The model under review builds one solid part; all positions refer to its coordinate system, in mm. A direction names the side the tool comes from. Round coordinates to 2 decimals unless told otherwise and drop trailing zeros. Loops run counter-clockwise (first coordinate to the right, second up) from the corner with the lowest first, then second, coordinate; pieces in that order, holes last. Notation, with made-up numbers: (-40, 5.25) -> (-1, 5.25) arc R23 ccw to (-1, 31.25) -> close; hole circle Ø6 at (56.5, 88). An arc over 180 degrees is marked (long way). Use a Markdown table: item, result. Add a question column.
1) Wall thickness on probe 1 along Z at (x, y) = (55, -17); probe 2 along Z at (x, y) = (34, -4.5); probe 3 along X at (y, z) = (-11.5, -120.65): over which ranges is each line inside the solid? List them lowest first.
2) Insertion check: pin 1 (5 mm diameter, centred on y = -13.5, z = -118, fed in from +X); pin 2 (1.5 mm diameter, centred on x = 8, z = -73, fed in from +Y); pin 3 (1 mm diameter, centred on x = 33, z = -109.5, fed in from -Y); pin 4 (8 mm diameter, centred on x = 8.5, z = -101, fed in from -Y). Each pin has a flat end and moves straight along its axis. Give the tip position at first contact, or say it passes through.
3) For faces 1 (the flat face through (36, -23, -137.16)), 2 (the flat face through (38, -23, -7.62)), 3 (the flat face through (38.5, 5.08, -53.3)), list the 3-axis set-ups (+Z, -Z, +X, -X, +Y, -Y) from which the entire face can be reached by the end or side of a thin tool; tool diameter is ignored.
4) Consider section A-A on z = -55.88. Give the boundary of the cut face in (x, y), plus the area to 3 significant figures.
5) Consider section C-C on z = -78.5. Give the boundary of the cut face in (x, y), plus the area to 3 significant figures.
6) Mouldability with a two-part tool opening along X and no side actions: class faces 4 (the cylindrical face through (41.156, 6.368, -61.832)), 5 (the flat face through (35, -23, 0)), 6 (the flat face through (0, -20, -69)) as released by +X, released by -X, zero draft, split by the parting line, or undercut.
7) Consider section D-D on x = 51. Give the boundary of the cut face in (y, z).
8) Consider section B-B on y = -24.13. Give the boundary of the cut face in (x, z).
from build123d import *

# Parameters (mm, degrees)
SKETCH1_W           = 58.42
SKETCH1_H           = 137.16
BOSS_EXTRUDE1_DEPTH = 7.62
SKETCH2_R           = 6.35
SKETCH2_R_2         = 4.826
BOSS_EXTRUDE2_DEPTH = 35.56
BOSS_EXTRUDE3_DEPTH = 35.56
FILLET1_R           = 19.05
FILLET2_R           = 12.7
BOSS_EXTRUDE4_DEPTH = 5.08
SKETCH7_R           = 7.5
CUT_EXTRUDE1_DEPTH  = 158.192964219
CUT_EXTRUDE2_START  = -5.08
SKETCH8_R           = 11
SKETCH8_R_2         = 7.5
CUT_EXTRUDE2_DEPTH  = 5.08
FILLET3_R           = 10.16
CUT_EXTRUDE3_REACH  = 157.273
SKETCH9_R           = 8.5


with BuildPart() as part:
    # Sketch1 → Boss-Extrude1 (new body)
    with BuildSketch(Plane(origin=(0, 0, 0), x_dir=(1, 0, 0), z_dir=(0, 1, 0))):
        with Locations((29.21, 68.58)):
            Rectangle(SKETCH1_W, SKETCH1_H)
    extrude(amount=BOSS_EXTRUDE1_DEPTH)

    # Sketch2 → Boss-Extrude2 (add)
    # profile 1 of 2: a face of its own
    with BuildSketch(Plane.XZ):
        with Locations(Location((28.448, -120.65, 0), (0, 0, 270))):
            Circle(SKETCH2_R)
        with Locations(Location((28.448, -120.65, 0), (0, 0, 270))):
            Circle(SKETCH2_R_2, mode=Mode.SUBTRACT)
    # profile 2 of 2: a face of its own
    with BuildSketch(Plane.XZ):
        with Locations(Location((28.448, -15.24, 0), (0, 0, 270))):
            Circle(SKETCH2_R)
        with Locations(Location((28.448, -15.24, 0), (0, 0, 270))):
            Circle(SKETCH2_R_2, mode=Mode.SUBTRACT)
    extrude(amount=BOSS_EXTRUDE2_DEPTH)

    # Sketch3 → Boss-Extrude3 (add)
    with BuildSketch(Plane.XZ):
        Polygon((58.42, -137.16), (0, -137.16), (0, 0), (58.42, 0), (58.42, -7.62), (7.62, -7.62), (7.62, -129.54), (58.42, -129.54), align=None)
    extrude(amount=BOSS_EXTRUDE3_DEPTH)

    # Fillet1
    fillet1_edges = [part.edges().sort_by_distance(p)[0] for p in [
        (29.21, 7.62, -137.16),
        (29.21, 7.62, 0),
    ]]
    fillet(fillet1_edges, radius=FILLET1_R)

    # Fillet2
    fillet2_edges = [part.edges().sort_by_distance(p)[0] for p in [
        (0, 7.62, -68.58),
        (0, -23.495, 0),
        (0, -23.495, -137.16),
        (0, 2.040384182, -131.580384182),
        (0, 2.040384182, -5.579615818),
    ]]
    fillet(fillet2_edges, radius=FILLET2_R)

    # Sketch4 → Boss-Extrude4 (add)
    with BuildSketch(Plane(origin=(58.42, 0, 0), x_dir=(0, 0, -1), z_dir=(1, 0, 0))):
        with BuildLine():
            Line((10.00175133, 5.334), (127.15824867, 5.334))
            ThreePointArc((127.15824867, 5.334), (122.77627796, 7.039660257), (118.11, 7.62))
            Line((118.11, 7.62), (19.05, 7.62))
            ThreePointArc((19.05, 7.62), (14.38372204, 7.039660257), (10.00175133, 5.334))
        make_face()
    extrude(amount=BOSS_EXTRUDE4_DEPTH)

    # Sketch7 → Cut-Extrude1 (cut, through all)
    with BuildSketch(Plane(origin=(0, 7.62, 0), x_dir=(1, 0, 0), z_dir=(0, 1, 0))):
        with Locations(Location((45.72, 55.88, 0), (0, 0, 270))):
            Circle(SKETCH7_R)
        with Locations(Location((33.02, 35.56, 0), (0, 0, 270))):
            Circle(SKETCH7_R)
    extrude(amount=-CUT_EXTRUDE1_DEPTH, mode=Mode.SUBTRACT)

    # Sketch8 → Cut-Extrude2 (cut)
    # profile 1 of 2: a face of its own
    with BuildSketch(Plane.XZ.offset(CUT_EXTRUDE2_START)):
        with Locations(Location((45.72, -55.88, 0), (0, 0, 270))):
            Circle(SKETCH8_R)
        with Locations(Location((45.72, -55.88, 0), (0, 0, 90))):
            Circle(SKETCH8_R_2, mode=Mode.SUBTRACT)
    # profile 2 of 2: a face of its own
    with BuildSketch(Plane.XZ.offset(CUT_EXTRUDE2_START)):
        with Locations(Location((33.02, -35.56, 0), (0, 0, 270))):
            Circle(SKETCH8_R)
        with Locations(Location((33.02, -35.56, 0), (0, 0, 90))):
            Circle(SKETCH8_R_2, mode=Mode.SUBTRACT)
    extrude(amount=CUT_EXTRUDE2_DEPTH, mode=Mode.SUBTRACT)

    # Fillet3
    # the kernel refuses this fillet: 10.16 mm, written as the material it adds along each edge
    with BuildSketch(Plane(origin=(17.78, -10.16, -119.38), x_dir=(0, 1, 0), z_dir=(-1, 0, 0))) as fillet3_piece_1_section:
        Polygon((0, 0), (FILLET3_R * 1.02, 0), (FILLET3_R * 1.02, FILLET3_R * 1.02), (0, FILLET3_R * 1.02), align=None)
    fillet3_piece_1 = extrude(amount=FILLET3_R * 1.02, mode=Mode.PRIVATE)
    fillet3_piece_1 = fillet3_piece_1 - Plane(origin=(17.78, -10.16, -119.38), x_dir=(0, -0.7071067811865475, 0.7071067811865475), z_dir=(-1, 0, 0)) * Sphere(FILLET3_R, mode=Mode.PRIVATE)
    add(fillet3_piece_1)
    with BuildSketch(Plane(origin=(17.78, -10.16, -17.78), x_dir=(0, 0, 1), z_dir=(-1, 0, 0))) as fillet3_piece_2_section:
        Polygon((0, 0), (FILLET3_R * 1.02, 0), (FILLET3_R * 1.02, FILLET3_R * 1.02), (0, FILLET3_R * 1.02), align=None)
    fillet3_piece_2 = extrude(amount=FILLET3_R * 1.02, mode=Mode.PRIVATE)
    fillet3_piece_2 = fillet3_piece_2 - Plane(origin=(17.78, -10.16, -17.78), x_dir=(0, -0.7071067811865475, -0.7071067811865475), z_dir=(-1, 0, 0)) * Sphere(FILLET3_R, mode=Mode.PRIVATE)
    add(fillet3_piece_2)
    with BuildSketch(Plane(origin=(17.78, 0, -129.54), x_dir=(0, 0, 1), z_dir=(1, 0, 0))) as fillet3_piece_3_section:
        with BuildLine():
            CenterArc((FILLET3_R, FILLET3_R), FILLET3_R, 180, 90)
            Line((0, FILLET3_R), (0, 0))
            Line((0, 0), (FILLET3_R, 0))
        make_face()
    fillet3_piece_3 = extrude(amount=40.64, mode=Mode.PRIVATE)
    fillet3_piece_3 = fillet3_piece_3 - Plane(origin=(28.448, -2.379056343, -120.65), x_dir=(0, 0, -1), z_dir=(0, 1, 0)) * Cylinder(4.826, 122, mode=Mode.PRIVATE)
    add(fillet3_piece_3)
    with BuildSketch(Plane(origin=(7.62, 0, -17.78), x_dir=(1, 0, 0), z_dir=(0, 0, -1))) as fillet3_piece_4:
        with BuildLine():
            CenterArc((FILLET3_R, FILLET3_R), FILLET3_R, 180, 90)
            Line((0, FILLET3_R), (0, 0))
            Line((0, 0), (FILLET3_R, 0))
        make_face()
    extrude(amount=101.6)
    with BuildSketch(Plane(origin=(7.62, -10.16, -129.54), x_dir=(1, 0, 0), z_dir=(0, -1, 0))) as fillet3_piece_5:
        with BuildLine():
            CenterArc((FILLET3_R, FILLET3_R), FILLET3_R, 180, 90)
            Line((0, FILLET3_R), (0, 0))
            Line((0, 0), (FILLET3_R, 0))
        make_face()
    extrude(amount=25.4)
    with BuildSketch(Plane(origin=(58.42, 0, -7.62), x_dir=(0, -1, 0), z_dir=(-1, 0, 0))) as fillet3_piece_6_section:
        with BuildLine():
            CenterArc((FILLET3_R, -FILLET3_R), FILLET3_R, 90, 90)
            Line((0, -FILLET3_R), (0, 0))
            Line((0, 0), (FILLET3_R, 0))
        make_face()
    fillet3_piece_6 = extrude(amount=40.64, mode=Mode.PRIVATE)
    fillet3_piece_6 = fillet3_piece_6 - Plane(origin=(28.448, -2.418481563, -15.24), x_dir=(0, 0, -1), z_dir=(0, 1, 0)) * Cylinder(4.826, 122, mode=Mode.PRIVATE)
    add(fillet3_piece_6)
    with BuildSketch(Plane(origin=(7.62, -10.16, -7.62), x_dir=(1, 0, 0), z_dir=(0, -1, 0))) as fillet3_piece_7:
        with BuildLine():
            CenterArc((FILLET3_R, -FILLET3_R), FILLET3_R, 90, 90)
            Line((0, -FILLET3_R), (0, 0))
            Line((0, 0), (FILLET3_R, 0))
        make_face()
    extrude(amount=25.4)

    # Sketch9 → Cut-Extrude3 (cut, up to next)
    with BuildSketch(Plane.ZY, mode=Mode.PRIVATE) as cut_extrude3_sk1:
        with Locations((-99.06, -24.13)):
            Circle(SKETCH9_R)
    cut_extrude3_tool1 = extrude(cut_extrude3_sk1.sketch, amount=-CUT_EXTRUDE3_REACH, mode=Mode.PRIVATE) & part.part
    add(cut_extrude3_tool1.solids().sort_by_distance((0, -24.13, -99.06))[0], mode=Mode.SUBTRACT)


solid = part.part
Result set:
| question | item | result |
|---|---|---|
| 1 | probe 1 | -137.16 to -129.54, -7.62 to 0 |
| 1 | probe 2 | -135.85 to -127.82, -123.73 to -117.57, -18.32 to -12.16, -9.34 to -1.31 |
| 1 | probe 3 | 0 to 7.7, 22.1 to 23.62, 33.27 to 34.8 |
| 2 | pin 1 | x = 34.8 |
| 2 | pin 2 | y = 6.99 |
| 2 | pin 3 | y = 0 |
| 2 | pin 4 | y = -35.56 |
| 3 | face 1 | -Z, +X, -X, +Y, -Y |
| 3 | face 2 | +X, -Y |
| 3 | face 3 | -Y |
| 4 | outline | (0, -35.56) -> (7.62, -35.56) -> (7.62, -10.16) arc R10.16 cw to (17.78, 0) -> (34.72, 0) -> (34.72, 5.08) -> (38.22, 5.08) -> (38.22, 7.62) -> (12.7, 7.62) arc R12.7 ccw to (0, -5.08) -> close; (53.22, 5.08) -> (56.72, 5.08) -> (56.72, 0) -> (58.42, 0) -> (58.42, 5.33) -> (63.5, 5.33) -> (63.5, 7.62) -> (53.22, 7.62) -> close |
| 4 | area | 565 mm2 |
| 5 | outline | (0, -35.56) -> (7.62, -35.56) -> (7.62, -10.16) arc R10.16 cw to (17.78, 0) -> (58.42, 0) -> (58.42, 5.33) -> (63.5, 5.33) -> (63.5, 7.62) -> (12.7, 7.62) arc R12.7 ccw to (0, -5.08) -> close |
| 5 | area | 715 mm2 |
| 6 | face 4 | undercut |
| 6 | face 5 | zero draft |
| 6 | face 6 | released by -X |
| 7 | outline | (-35.56, -137.16) -> (-11.43, -137.16) arc R19.05 ccw to (7.62, -118.11) -> (7.62, -61.21) -> (5.08, -61.21) -> (5.08, -65.53) -> (0, -65.53) -> (0, -119.38) arc R10.16 cw to (-10.16, -129.54) -> (-35.56, -129.54) -> close; (-35.56, -7.62) -> (-10.16, -7.62) arc R10.16 cw to (0, -17.78) -> (0, -46.23) -> (5.08, -46.23) -> (5.08, -50.55) -> (7.62, -50.55) -> (7.62, -19.05) arc R19.05 ccw to (-11.43, 0) -> (-35.56, 0) -> close |
| 8 | outline | (0, -124.46) arc R12.7 ccw to (12.7, -137.16) -> (58.42, -137.16) -> (58.42, -129.54) -> (17.78, -129.54) arc R10.16 cw to (7.62, -119.38) -> (7.62, -107.56) -> (0, -107.56) -> close; (0, -90.56) -> (7.62, -90.56) -> (7.62, -17.78) arc R10.16 cw to (17.78, -7.62) -> (58.42, -7.62) -> (58.42, 0) -> (12.7, 0) arc R12.7 ccw to (0, -12.7) -> close; circle Ø12.7 at (28.45, -120.65); circle Ø12.7 at (28.45, -15.24); hole circle Ø9.65 at (28.45, -120.65); hole circle Ø9.65 at (28.45, -15.24) |
